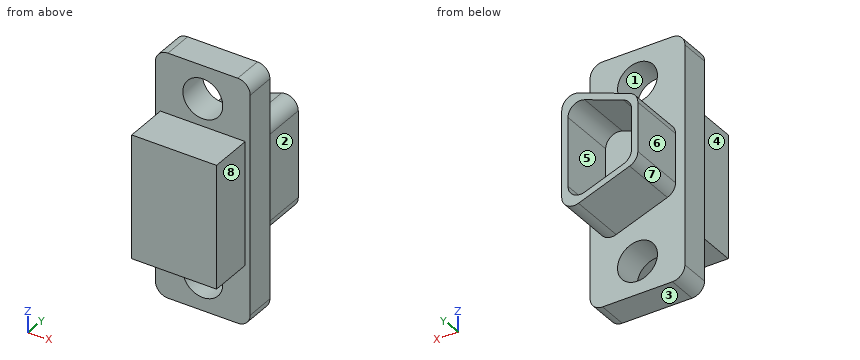
Autodesk Inventor part; units mm, degrees
ref_plane "YZ Plane" through (0, 0, 0) normal (1, 0, 0) x (0, 1, 0)
ref_plane "XZ Plane" through (0, 0, 0) normal (0, 1, 0) x (-1, 0, 0)
ref_plane "XY Plane" through (0, 0, 0) normal (0, 0, 1) x (1, 0, 0)
sketch "Sketch1" plane through (0, 0, 0) normal (0, 1, 0) x (-1, 0, 0)
  line L0 (3.8, 9.8) -> (-3.8, 9.8)
  line L1 (-3.8, 9.8) -> (-3.8, -9.8)
  line L2 (-3.8, -9.8) -> (3.8, -9.8)
  line L3 (3.8, -9.8) -> (3.8, 9.8)
  circle A0 centre (0, 7.15) radius 1.6
  circle A1 centre (0, -7.15) radius 1.6
  point P0 (0, 0)
  dimension "d0" = 19.6
  dimension "d1" = 7.6
  dimension "d2" = 9.8
  dimension "d3" = 3.8
  dimension "d4" = 3.2
  dimension "d5" = 3.2
  dimension "d6" = 14.3
  dimension "d7" = 7.15
extrude "Extrusion1" add sketch "Sketch1" along normal blind 2.4
fillet "Fillet1" radius 1 4 edges at (3.8, 1.2, 9.8) (-3.8, 1.2, 9.8) (3.8, 1.2, -9.8) (-3.8, 1.2, -9.8)
sketch "Sketch2" plane through (0, 2.4, 0) normal (0, 1, 0) x (1, 0, 0)
  line L0 (-3.05, -2.6694) -> (-3.05, 2.6694)
  line L1 (-3.05, 2.6694) -> (3.05, 4.9)
  line L2 (3.05, 4.9) -> (3.05, -4.9)
  line L3 (3.05, -4.9) -> (-3.05, -2.6694)
  line L4 (2.55, -4.1848) -> (-2.55, -2.3198)
  line L5 (-2.55, -2.3198) -> (-2.55, 2.3198)
  line L6 (-2.55, 2.3198) -> (2.55, 4.1848)
  line L7 (2.55, 4.1848) -> (2.55, -4.1848)
  point P0 (0, 0)
  dimension "d11" = 69.914
  dimension "d13" = 9.8
  dimension "d14" = 6.1
  dimension "d15" = 3.05
  dimension "d17" = 0.5
  dimension "d18" = 0.5
  dimension "d19" = 0.5
  dimension "d20" = 0.5
  dimension "d21" = 4.9
  dimension "d22" = 69.914
  dimension "d23" = 69.914
extrude "Extrusion2" add sketch "Sketch2" along normal blind 4.6
fillet "Fillet2" radius 1 8 edges at (-3.05, 4.7, -2.6694) (-3.05, 4.7, 2.6694) (3.05, 4.7, 4.9) (3.05, 4.7, -4.9) (-2.55, 4.7, -2.3198) (-2.55, 4.7, 2.3198) (2.55, 4.7, -4.1848) (2.55, 4.7, 4.1848)
sketch "Sketch3" plane through (0, 0, 0) normal (0, -1, 0) x (1, 0, 0)
  line L0 (3.4, 4.95) -> (-3.4, 4.95)
  line L1 (-3.4, 4.95) -> (-3.4, -4.95)
  line L2 (-3.4, -4.95) -> (3.4, -4.95)
  line L3 (3.4, -4.95) -> (3.4, 4.95)
  point P0 (0, 0)
  dimension "d27" = 9.9
  dimension "d28" = 6.8
  dimension "d29" = 4.95
  dimension "d30" = 3.4
extrude "Extrusion3" add sketch "Sketch3" along normal blind 3.5
equation "\"d5\" = d4"
equation "\"d22\" = d11"
properties part number "9pin female connector"
Can you work these out from the model? Positions are in its coordinate system, mm. Face numbers are marked on the shaded views. A direction names the side the tool comes from. Give positions to 0.01 mm unless a question says otherwise; leave off trailing zeros. Write each loop counter-clockwise with the first axis right and the second up, starting at its lowest first coordinate (ties: lowest second). Pieces come first, ordered by that corner, then holes. Notation, with made-up numbers: (-33, 88) -> (-1, 88) arc R20 ccw to (-1, 92) -> close; hole circle Ø6 at (9, 87.25). An arc over 180 degrees is marked (long way). Answer as a JSON object with one key per item and string values. Group by question number.
Item 1: Suppose I cut it at D-D (y = -0.25). Please give me the cut outline in (x, z).
Item 2: Suppose I cut it at C-C (z = 0.25). Please give me the cut outline in (x, y), plus the area to 3 significant figures.
Item 3: Please list where these lines run through material, in increasing order: line 1 (Z direction, x = 0, y = 1.05); line 2 (Y direction, x = 1.25, z = 8.75); line 3 (Z direction, x = -0.75, y = 1). Write a range as [from, to].
Item 4: Suppose I cut it at A-A (z = -7.15). Please give me the cut outline in (x, y), plus the area to 3 significant figures.
Item 5: I'm going to push flat-ended pins straight in: P1, Ø2.5, axis at y = 4, z = -0.5, coming from the +X side; P2, Ø1, axis at x = -0.5, y = -1, coming from the +Z side; P3, Ø1.2, axis at y = 4, z = -1, coming from the -X side; P4, Ø1.9, axis at x = 0, z = 7.15, coming from the +Y side. Where does each tip first touch, or does it pass through?
Item 6: For the marked faces 5, 6, 7 and 8, which set-ups out of +Z, -Z, +X, -X, +Y, -Y let a thin tool reach every point of the face, with its end or its side?
Item 7: Suppose I cut it at B-B (x = 0.25). Please give me the cut outline in (y, z).
Item 8: We'd pull the mould along X, two halves only. Please class the marked faces 1, 2, 3 and 4: +X half, -X half, draft (parallel to the pull), parting line (faces both ways), or undercut.
Findings:
{
 "1": {"outline": "(-3.4, -4.95) -> (3.4, -4.95) -> (3.4, 4.95) -> (-3.4, 4.95) -> close"},
 "2": {"outline": "(-3.8, 0) -> (-3.4, 0) -> (-3.4, -3.5) -> (3.4, -3.5) -> (3.4, 0) -> (3.8, 0) -> (3.8, 2.4) -> (3.05, 2.4) -> (3.05, 7) -> (2.55, 7) -> (2.55, 2.4) -> (-2.55, 2.4) -> (-2.55, 7) -> (-3.05, 7) -> (-3.05, 2.4) -> (-3.8, 2.4) -> close", "area": "46.6 mm²"},
 "3": {"line 1": "z = [-9.8, -8.75], [-5.55, 5.55], [8.75, 9.8]", "line 2": "y = [0, 2.4]", "line 3": "z = [-9.8, -8.56], [-5.74, 5.74], [8.56, 9.8]"},
 "4": {"outline": "(-3.8, 0) -> (-1.6, 0) -> (-1.6, 2.4) -> (-3.8, 2.4) -> close; (1.6, 0) -> (3.8, 0) -> (3.8, 2.4) -> (1.6, 2.4) -> close", "area": "10.6 mm²"},
 "5": {"P1": "stops at x = 3.05", "P2": "stops at z = 4.95", "P3": "stops at x = -3.05", "P4": "passes through"},
 "6": {"face 5": "+Y", "face 6": "+Z, -Z, -X, +Y", "face 7": "-Z, -X, +Y", "face 8": "+Z, -Z, +X, -Y"},
 "7": {"outline": "(-3.5, -4.95) -> (0, -4.95) -> (0, -5.57) -> (2.4, -5.57) -> (2.4, -3.88) -> (7, -3.88) -> (7, -3.34) -> (2.4, -3.34) -> (2.4, 3.34) -> (7, 3.34) -> (7, 3.88) -> (2.4, 3.88) -> (2.4, 5.57) -> (0, 5.57) -> (0, 4.95) -> (-3.5, 4.95) -> close; (0, -9.8) -> (2.4, -9.8) -> (2.4, -8.73) -> (0, -8.73) -> close; (0, 8.73) -> (2.4, 8.73) -> (2.4, 9.8) -> (0, 9.8) -> close"},
 "8": {"face 1": "undercut", "face 2": "+X half", "face 3": "draft", "face 4": "-X half"}
}
